```python
from build123d import *

# Parameters (mm, degrees)
SKETCH3_R            = 12.7
BOSS_EXTRUDE1_DEPTH  = 76.2
BOSS_EXTRUDE2_DEPTH  = 6.35
SKETCH6_W            = 63.5
SKETCH6_H            = 50.8
BOSS_EXTRUDE3_DEPTH  = 6.35
SKETCH9_W            = 50.8
SKETCH9_H            = 6.35
BOSS_EXTRUDE4_DEPTH  = 0.38862
SKETCH10_W           = 0.38862
SKETCH10_H           = 50.8
BOSS_EXTRUDE5_DEPTH  = 25.4
SKETCH11_W           = 50.8
SKETCH11_H           = 6.35
BOSS_EXTRUDE6_DEPTH  = 0.38862
SKETCH13_W           = 0.38862
SKETCH13_H           = 50.8
BOSS_EXTRUDE7_DEPTH  = 25.4
SKETCH14_W           = 0.38862
SKETCH14_H           = 50.8
BOSS_EXTRUDE8_DEPTH  = 10.8712
SKETCH15_W           = 50.8
SKETCH15_H           = 10.8712
BOSS_EXTRUDE9_DEPTH  = 25.76322
SKETCH16_W           = 0.38862
SKETCH16_H           = 50.8
BOSS_EXTRUDE10_DEPTH = 10.8712
SKETCH17_W           = 50.8
SKETCH17_H           = 10.8712
BOSS_EXTRUDE11_DEPTH = 25.76322
RIB4_REACH           = 127.041
SKETCH21_WALL_W      = 279.8678728
SKETCH21_WALL_H      = 25.4
RIB15_REACH          = 127.041
SKETCH22_WALL_W      = 278.64922185
SKETCH22_WALL_H      = 25.4
SKETCH26_W           = 25.4
SKETCH26_H           = 12.600318116
BOSS_EXTRUDE12_DEPTH = 44.45
SKETCH27_W           = 50.8
SKETCH27_H           = 42.6212
BOSS_EXTRUDE13_DEPTH = 6.35
SKETCH28_W           = 50.8
SKETCH28_H           = 42.6212
BOSS_EXTRUDE14_DEPTH = 6.35


with BuildPart() as part:
    # Sketch3 → Boss-Extrude1 (new body)
    with BuildSketch(Plane.XY):
        with Locations(Location((0, 0, 0), (0, 0, 180))):
            Circle(SKETCH3_R)
    extrude(amount=BOSS_EXTRUDE1_DEPTH)

    # Sketch4 → Boss-Extrude2 (add)
    with BuildSketch(Plane(origin=(0, 0, 0), x_dir=(-1, 0, 0), z_dir=(0, 0, -1))):
        Polygon((0, 0), (19.05, 0), (19.05, 50.8), (-19.05, 50.8), (-19.05, 0), align=None)
    extrude(amount=-BOSS_EXTRUDE2_DEPTH)

    # Sketch6 → Boss-Extrude3 (add)
    with BuildSketch(Plane(origin=(0, 50.8, 0), x_dir=(1, 0, 0), z_dir=(0, 1, 0))):
        with Locations((1.04805825, -17.613482739)):
            Rectangle(SKETCH6_W, SKETCH6_H)
    extrude(amount=BOSS_EXTRUDE3_DEPTH)

    # Sketch9 → Boss-Extrude4 (add)
    with BuildSketch(Plane(origin=(32.79805825, 0, 0), x_dir=(0, 0, -1), z_dir=(1, 0, 0))):
        with Locations((-17.613482739, 53.975)):
            Rectangle(SKETCH9_W, SKETCH9_H)
    extrude(amount=BOSS_EXTRUDE4_DEPTH)

    # Sketch10 → Boss-Extrude5 (add)
    with BuildSketch(Plane(origin=(0, 57.15, 0), x_dir=(1, 0, 0), z_dir=(0, 1, 0))):
        with Locations((32.99236825, -17.613482739)):
            Rectangle(SKETCH10_W, SKETCH10_H)
    extrude(amount=BOSS_EXTRUDE5_DEPTH)

    # Sketch11 → Boss-Extrude6 (add)
    with BuildSketch(Plane.ZY.offset(30.70194175)):
        with Locations((17.613482739, 53.975)):
            Rectangle(SKETCH11_W, SKETCH11_H)
    extrude(amount=BOSS_EXTRUDE6_DEPTH)

    # Sketch13 → Boss-Extrude7 (add)
    with BuildSketch(Plane(origin=(0, 57.15, 0), x_dir=(1, 0, 0), z_dir=(0, 1, 0))):
        with Locations((-30.89625175, -17.613482739)):
            Rectangle(SKETCH13_W, SKETCH13_H)
    extrude(amount=BOSS_EXTRUDE7_DEPTH)

    # Sketch14 → Boss-Extrude8 (add)
    with BuildSketch(Plane(origin=(0, 82.55, 0), x_dir=(1, 0, 0), z_dir=(0, 1, 0))):
        with Locations((-30.89625175, -17.613482739)):
            Rectangle(SKETCH14_W, SKETCH14_H)
    extrude(amount=BOSS_EXTRUDE8_DEPTH)

    # Sketch15 → Boss-Extrude9 (add)
    with BuildSketch(Plane(origin=(-30.70194175, 0, 0), x_dir=(0, 0, -1), z_dir=(1, 0, 0))):
        with Locations((-17.613482739, 87.9856)):
            Rectangle(SKETCH15_W, SKETCH15_H)
    extrude(amount=BOSS_EXTRUDE9_DEPTH)

    # Sketch16 → Boss-Extrude10 (add)
    with BuildSketch(Plane(origin=(0, 82.55, 0), x_dir=(1, 0, 0), z_dir=(0, 1, 0))):
        with Locations((32.99236825, -17.613482739)):
            Rectangle(SKETCH16_W, SKETCH16_H)
    extrude(amount=BOSS_EXTRUDE10_DEPTH)

    # Sketch17 → Boss-Extrude11 (add)
    with BuildSketch(Plane.ZY.offset(-32.79805825)):
        with Locations((17.613482739, 87.9856)):
            Rectangle(SKETCH17_W, SKETCH17_H)
    extrude(amount=BOSS_EXTRUDE11_DEPTH)

    # Sketch21 wall → Rib4 (add, up to next)
    with BuildSketch(Plane(origin=(0, 38.1, 11.981741369), x_dir=(0, 0.914150584151, 0.405374776592), z_dir=(0, -0.405374776592, 0.914150584151)), mode=Mode.PRIVATE) as rib4_sk1:
        Rectangle(SKETCH21_WALL_W, SKETCH21_WALL_H)
    rib4_tool1 = extrude(rib4_sk1.sketch, amount=-RIB4_REACH, mode=Mode.PRIVATE) - part.part
    add(rib4_tool1.solids().sort_by_distance((0, 38.1, 11.981741369))[0])

    # Sketch22 wall → Rib15 (add, up to next)
    with BuildSketch(Plane(origin=(0, 38.1, -3.893258631), x_dir=(0, 0.956083915685, -0.293093067419), z_dir=(0, 0.293093067419, 0.956083915685)), mode=Mode.PRIVATE) as rib15_sk1:
        Rectangle(SKETCH22_WALL_W, SKETCH22_WALL_H)
    rib15_tool1 = extrude(rib15_sk1.sketch, amount=RIB15_REACH, mode=Mode.PRIVATE) - part.part
    add(rib15_tool1.solids().sort_by_distance((0, 38.1, -3.893258631))[0])

    # Sketch26 → Boss-Extrude12 (add)
    with BuildSketch(Plane(origin=(0, 50.8, 0), x_dir=(-1, 0, 0), z_dir=(0, -1, 0))):
        with Locations((0, -36.713323681)):
            Rectangle(SKETCH26_W, SKETCH26_H)
    extrude(amount=BOSS_EXTRUDE12_DEPTH)

    # Sketch27 → Boss-Extrude13 (add)
    with BuildSketch(Plane(origin=(33.18667825, 0, 0), x_dir=(0, 0, -1), z_dir=(1, 0, 0))):
        with Locations((-17.613482739, 72.1106)):
            Rectangle(SKETCH27_W, SKETCH27_H)
    extrude(amount=BOSS_EXTRUDE13_DEPTH)

    # Sketch28 → Boss-Extrude14 (add)
    with BuildSketch(Plane.ZY.offset(31.09056175)):
        with Locations((17.613482739, 72.1106)):
            Rectangle(SKETCH28_W, SKETCH28_H)
    extrude(amount=BOSS_EXTRUDE14_DEPTH)


solid = part.part
```
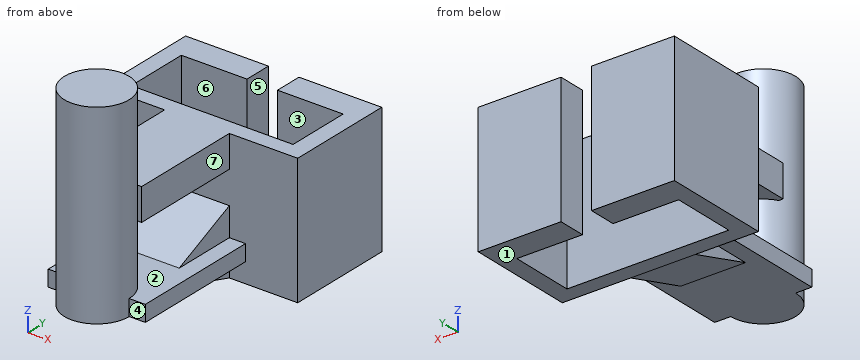
For this review, take the finished solid that the model builds, in its own axes (mm). Face numbers are marked on the shaded views. A direction names the side the tool comes from. Give positions to 0.01 mm unless a question says otherwise; leave off trailing zeros. Write each loop counter-clockwise with the first axis right and the second up, starting at its lowest first coordinate (ties: lowest second). Pieces come first, ordered by that corner, then holes.
Item 1: Wall thickness on probe 1 along Y at (x, z) = (-29, 19); probe 2 along X at (y, z) = (78.5, 33); probe 3 along Z at (x, y) = (-15, 47): over which ranges is each line inside the solid? List them lowest first.
Item 2: Take a section at D-D (z = 2). Give the boundary of the cut face in (x, y), and give its area (3 significant figures).
Item 3: Machinability: for the marked faces 4, 5, 6 and 7, which of the approach directions +Z, -Z, +X, -X, +Y, -Y give a long, thin tool a straight path to every point of the face, cutting with its end or side? Answer none if there is none.
Item 4: Take a section at B-B (z = 29). Give the boundary of the cut face in (x, y), and give its area (3 significant figures).
Item 5: The part is to be moulded in two halves that separate along Z. For the marked faces 1, 2 and 3, say which applies: +Z half, -Z half, draft (parallel to the pull), parting line (faces both ways), or undercut.
Item 6: Take a section at A-A (x = 0). Give the boundary of the cut face in (y, z).
Item 7: Insertion check: P1, Ø3, axis at x = 16.5, z = 1.5, coming from the -Y side; P2, Ø3, axis at y = 31.5, z = 3.5, coming from the -X side; P3, Ø20.5, axis at x = -1.5, y = 25, coming from the -Z side. Each pin has a flat end and moves straight along its axis. Give the tip position at first contact, or say it passes through.
Item 8: Take a section at C-C (x = 17). Give the boundary of the cut face in (y, z), and give its area (3 significant figures).
Established:
1. probe 1: y = 50.8 to 57.15, 82.55 to 93.42
1. probe 2: x = -37.44 to -30.7, 32.8 to 39.54
1. probe 3: z = 0 to 6.35
2. outline: (-37.44, 50.8) - (-19.05, 50.8) - (-19.05, 0) - (-12.7, 0) arc R12.7 ccw to (12.7, 0) - (19.05, 0) - (19.05, 50.8) - (39.54, 50.8) - (39.54, 93.42) - (7.03, 93.42) - (7.03, 82.55) - (32.8, 82.55) - (32.8, 57.15) - (-30.7, 57.15) - (-30.7, 82.55) - (-4.94, 82.55) - (-4.94, 93.42) - (-37.44, 93.42) - close
2. area: 3,730 mm2
3. face 4: +Z, -Z, +X, -Y
3. face 5: +Z, -Z, +Y
3. face 6: +Z, -Z
3. face 7: +Z, +X, -Y
4. outline: (-37.44, 50.8) - (39.54, 50.8) - (39.54, 93.42) - (7.03, 93.42) - (7.03, 82.55) - (32.8, 82.55) - (32.8, 57.15) - (-30.7, 57.15) - (-30.7, 82.55) - (-4.94, 82.55) - (-4.94, 93.42) - (-37.44, 93.42) - close; circle Ø25.4 at (0, 0)
4. area: 2,040 mm2
5. face 1: -Z half
5. face 2: undercut
5. face 3: draft
6. outline: (-12.7, 0) - (25.4, 0) - (50.8, -7.79) - (57.15, -7.79) - (57.15, 43.01) - (12.7, 43.01) - (12.7, 76.2) - (-12.7, 76.2) - close; hole (12.7, 6.35) - (25.4, 6.35) - (50.8, 17.61) - (50.8, 30.41) - (12.7, 30.41) - close
7. P1: stops at y = 0
7. P2: stops at x = -19.05
7. P3: stops at z = -3.02
8. outline: (0, 0) - (50.8, 0) - (50.8, -7.79) - (57.15, -7.79) - (57.15, 43.01) - (50.8, 43.01) - (50.8, 6.35) - (0, 6.35) - close; (82.55, -7.79) - (93.42, -7.79) - (93.42, 43.01) - (82.55, 43.01) - close
8. area: 1,200 mm2
